Check sheet for the drawn part. Datum: minimum x, y, z corner. Units: mm. Round coordinates to 2 decimals unless told otherwise and drop trailing zeros. Write each loop counter-clockwise with the first axis right and the second up, starting at its lowest first coordinate (ties: lowest second). Pieces come first, ordered by that corner, then holes. Notation, with made-up numbers: (-36, -15.75) - (-9, -15.75) arc R15 ccw to (-9, 11.25) - close; hole circle Ø10 at (66.5, 22.5). An arc over 180 degrees is marked (long way). Return JSON: item names as keys, results as strings. Group by question number.
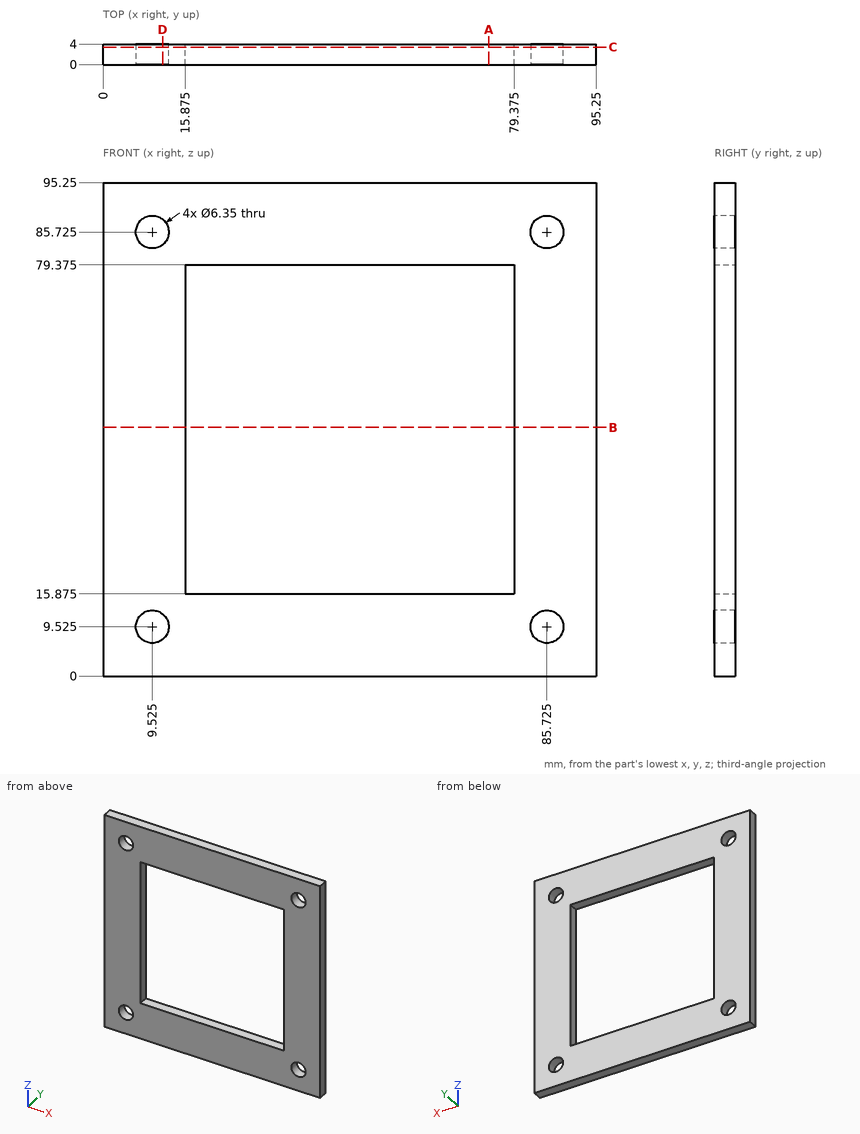
1. Section check A-A (x = 74.5). Enter the section's corners in (y, z) (3 decimals), and give its area (3 significant figures).
2. Section check C-C (y = 3.4). Enter the section's corners in (x, z) (3 decimals).
3. Section check B-B (z = 48). Enter the section's corners in (x, y) (3 decimals).
4. Material ranges on line 1 along Z through (x, y) = (86, 2.4); line 2 along X through (y, z) = (3.15, 19) (3 decimals), recorded low to high.
5. Section check D-D (x = 11.5). Enter the section's corners in (y, z).
Result sheet:
{
 "1": {"outline": "(0, 0) - (4, 0) - (4, 15.875) - (0, 15.875) - close; (0, 79.375) - (4, 79.375) - (4, 95.25) - (0, 95.25) - close", "area": "127 mm²"},
 "2": {"outline": "(0, 0) - (95.25, 0) - (95.25, 95.25) - (0, 95.25) - close; hole circle Ø6.35 at (9.525, 9.525); hole circle Ø6.35 at (9.525, 85.725); hole (15.875, 15.875) - (79.375, 15.875) - (79.375, 79.375) - (15.875, 79.375) - close; hole circle Ø6.35 at (85.725, 9.525); hole circle Ø6.35 at (85.725, 85.725)"},
 "3": {"outline": "(0, 0) - (15.875, 0) - (15.875, 4) - (0, 4) - close; (79.375, 0) - (95.25, 0) - (95.25, 4) - (79.375, 4) - close"},
 "4": {"line 1": "z = 0 to 6.36, 12.69 to 82.56, 88.89 to 95.25", "line 2": "x = 0 to 15.875, 79.375 to 95.25"},
 "5": {"outline": "(0, 0) - (4, 0) - (4, 7.04) - (0, 7.04) - close; (0, 12.01) - (4, 12.01) - (4, 83.24) - (0, 83.24) - close; (0, 88.21) - (4, 88.21) - (4, 95.25) - (0, 95.25) - close"}
}
